Geometry: final body of the model. Coordinates: model frame, mm. Face numbers are marked on the shaded views. A direction names the side the tool comes from. Give positions to 0.01 mm unless a question says otherwise; leave off trailing zeros. Order: outer loops, then holes, each group sorted by start corner. A loop starts at its lowest first (then second) coordinate and runs counter-clockwise, first axis right, second up. Notation, with made-up numbers: (-29, 45.5) -> (21, 45.5) arc R7 cw to (21, 50.5) -> close; hole circle Ø3 at (-10.5, -25.75). An arc over 180 degrees is marked (long way). One line per question, with ' | ' between items. Start each with the question number.
(1) Ray query, L1, parallel to Z at x = -17.25, y = 18.75; L2, parallel to Z at x = -14.75, y = 10.25; L3, parallel to Y at x = -9, z = 21. Return the intervals inside material, ascending.
(2) Section A-A (z = 18.75). Return loops of the section in (x, y).
(3) First-contact query: pin 1 Ø4 at (x, z) = (-11, 20.5) entering from +Y; pin 2 Ø2.5 at (x, z) = (-11, 18) entering from -Y; pin 3 Ø1.5 at (y, z) = (5.5, 10.5) entering from -X; pin 4 Ø6 at (x, z) = (-18.5, 18) entering from -Y. Flat tips, straight axial feed; report the tip coordinate or a pass-through.
(4) Mould query, pull axis Y, two halves, no side actions, for the marked faces 1, 2, 3 and 4. Classes: +Y half, -Y half, draft (parallel to the pull), parting line (faces both ways), or undercut.
(5) Section B-B (x = -11.25). Return loops of the section in (y, z).
(6) Set-up query: the marked faces 5, 6, 7, 8 and 9. Return all of +Z, -Z, +X, -X, +Y, -Y with unobstructed straight access to the full face (end or side cutting, diameter ignored); none if empty.
(7) Section C-C (y = 12.75). Return loops of the section in (x, z), then the cut area to 3 significant figures.
(8) Section D-D (z = 21.5). Return loops of the section in (x, y), then the cut area to 3 significant figures.
Autodesk Inventor part; units mm, degrees
ref_plane "YZ Plane" through (0, 0, 0) normal (1, 0, 0) x (0, 1, 0)
ref_plane "XZ Plane" through (0, 0, 0) normal (0, 1, 0) x (-1, 0, 0)
ref_plane "XY Plane" through (0, 0, 0) normal (0, 0, 1) x (1, 0, 0)
ref_plane "Work Plane1" through (-10.8248, 8.3603, 0) normal (0, 0, 1) x (1, 0, 0)
sketch "Sketch3" plane through (-10.8248, 8.3603, 0) normal (0, 0, 1) x (1, 0, 0)
  circle A0 centre (0, 0) radius 12
  point P0 (0, 0)
  dimension "d0" = 24
extrude "Extrusion1" add sketch "Sketch3" along normal blind 1
sketch "Sketch4" plane through (-10.8248, 8.3603, 1) normal (0, 0, 1) x (1, 0, 0)
  circle A0 centre (0, 0) radius 13
  circle A1 centre (0, 0) radius 12
  dimension "d4" = 26
extrude "Extrusion2" add sketch "Sketch4" along normal blind 12 contours A0 | A1
sketch "Sketch5" plane through (-10.8248, 8.3603, 13) normal (0, 0, 1) x (1, 0, 0)
  line L0 (-3.81, 2.1338) -> (3.81, 2.1338)
  line L1 (3.81, 2.1338) -> (3.81, 5.3088)
  line L2 (3.81, 5.3088) -> (-3.81, 5.3088)
  line L3 (-3.81, 5.3088) -> (-3.81, 2.1338)
  line L4 (-3.81, -4.2162) -> (3.81, -4.2162)
  line L5 (3.81, -4.2162) -> (3.81, -1.0412)
  line L6 (3.81, -1.0412) -> (-3.81, -1.0412)
  line L7 (-3.81, -1.0412) -> (-3.81, -4.2162)
  circle A0 centre (0, 0) radius 13
  point P0 (0, -7.7939)
  dimension "d15" = 7.62
  dimension "d16" = 3.175
  dimension "d17" = 7.62
  dimension "d18" = 3.175
  dimension "d19" = 3.175
  dimension "d20" = 3.81
  dimension "d21" = 3.81
extrude "Extrusion3" add sketch "Sketch5" along normal blind 12 contours L3 L2 L1 L0 | L7 L6 L5 L4
sketch "Sketch6" plane through (-15.5873, 4.1441, 13) normal (0, -1, 0) x (1, 0, 0)
  circle A0 centre (4.7625, 7.9375) radius 1.5685
  line L0 (0.9525, 0) -> (0.9525, 12)
  point P0 (4.7625, -37.7)
  dimension "d22" = 3.81
extrude "Extrusion4" cut sketch "Sketch6" against normal blind 12
properties part number "Swing_Joint_2"
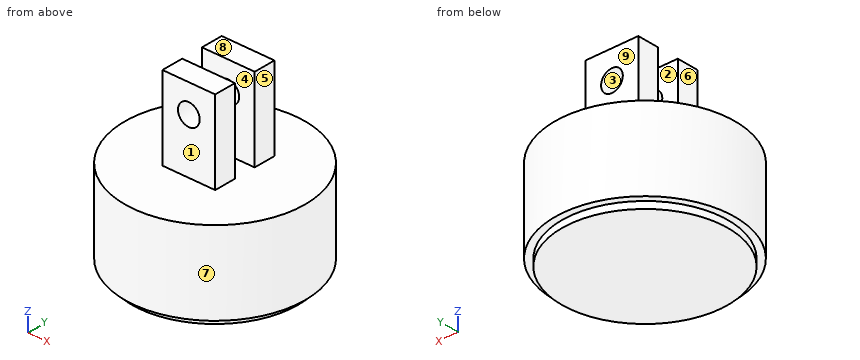
Response:
1) L1: z = 1 to 13 | L2: z = 0 to 13 | L3: y = 4.14 to 7.32, 10.49 to 13.67
2) outline: (-14.63, 4.14) -> (-7.01, 4.14) -> (-7.01, 7.32) -> (-14.63, 7.32) -> close; (-14.63, 10.49) -> (-7.01, 10.49) -> (-7.01, 13.67) -> (-14.63, 13.67) -> close
3) pin 1: stops at y = 13.67 | pin 2: stops at y = 4.14 | pin 3: stops at x = -23.65 | pin 4: passes through
4) face 1: -Y half | face 2: undercut | face 3: draft | face 4: undercut
5) outline: (-4.63, 1) -> (-3.63, 1) -> (-3.63, 0) -> (20.35, 0) -> (20.35, 1) -> (21.35, 1) -> (21.35, 13) -> (13.67, 13) -> (13.67, 19.43) -> (10.49, 19.43) -> (10.49, 13) -> (7.32, 13) -> (7.32, 19.43) -> (4.14, 19.43) -> (4.14, 13) -> (-4.63, 13) -> close; (4.14, 22.45) -> (7.32, 22.45) -> (7.32, 25) -> (4.14, 25) -> close; (10.49, 22.45) -> (13.67, 22.45) -> (13.67, 25) -> (10.49, 25) -> close
6) face 5: +Z, +X, +Y, -Y | face 6: +Z, -X, +Y, -Y | face 7: +Z, -Z | face 8: +Z, +X, -X, +Y, -Y | face 9: +Z, +X, -X, +Y
7) outline: (-23.06, 1) -> (-21.99, 1) -> (-21.99, 0) -> (0.34, 0) -> (0.34, 1) -> (1.41, 1) -> (1.41, 13) -> (-7.01, 13) -> (-7.01, 25) -> (-14.63, 25) -> (-14.63, 13) -> (-23.06, 13) -> close; hole circle Ø3.14 at (-10.82, 20.94) | area: 400 mm^2
8) outline: (-14.63, 4.14) -> (-12.29, 4.14) -> (-12.29, 7.32) -> (-14.63, 7.32) -> close; (-14.63, 10.49) -> (-12.29, 10.49) -> (-12.29, 13.67) -> (-14.63, 13.67) -> close; (-9.36, 4.14) -> (-7.01, 4.14) -> (-7.01, 7.32) -> (-9.36, 7.32) -> close; (-9.36, 10.49) -> (-7.01, 10.49) -> (-7.01, 13.67) -> (-9.36, 13.67) -> close | area: 29.8 mm^2
